```python
from build123d import *

# Parameters (mm, degrees)
PAD_DEPTH       = 33
POCKET_DEPTH    = 28
PAD001_DEPTH    = 4
SKETCH003_R     = 2.75
PAD002_DEPTH    = 5
SKETCH004_R     = 3.125
PAD003_DEPTH    = 3
FILLET_R        = 34
FILLET001_R     = 12
FILLET002_R     = 2
CHAMFER_SIZE    = 1
CHAMFER001_SIZE = 1
CHAMFER002_SIZE = 1


with BuildPart() as part:
    # Sketch → Pad (new body)
    with BuildSketch(Plane.XY):
        Polygon((-30, 0), (30, 0), (30, -51.038384), (0, -120), (-30, -51.038384), align=None)
    extrude(amount=PAD_DEPTH)

    # Sketch001 (on Face7 of Pad) → Pocket (cut)
    with BuildSketch(Plane.XY.offset(33)):
        Polygon((-22.25, 3.29609), (22.25, 3.29609), (22.25, -49.798735), (0, -100), (-22.25, -49.798735), align=None)
    extrude(amount=-POCKET_DEPTH, mode=Mode.SUBTRACT)

    # Sketch002 (on Face4 of Pocket) → Pad001 (join)
    with BuildSketch(Plane.XY.offset(33)):
        Polygon((-30, 0), (30, 0), (30, -51.038384), (0, -120), (-30, -51.038384), align=None)
    extrude(amount=-PAD001_DEPTH)

    # Sketch003 (on Face2 of Pad001) → Pad002 (join)
    with BuildSketch(Plane(origin=(0, 0, 0), x_dir=(1, 0, 0), z_dir=(0, 0, -1))):
        with Locations((-12.7, 22.314992)):
            Circle(SKETCH003_R)
        with Locations((12.7, 22.314992)):
            Circle(SKETCH003_R)
        with Locations((-12.7, 47.714992)):
            Circle(SKETCH003_R)
        with Locations((12.7, 47.714992)):
            Circle(SKETCH003_R)
    extrude(amount=PAD002_DEPTH)

    # Sketch004 (on Face25 of Pad002) → Pad003 (join)
    with BuildSketch(Plane(origin=(0, 0, -5), x_dir=(1, 0, 0), z_dir=(0, 0, -1))):
        with Locations((12.7, 47.714992)):
            Circle(SKETCH004_R)
        with Locations((-12.7, 47.714992)):
            Circle(SKETCH004_R)
        with Locations((-12.7, 22.314992)):
            Circle(SKETCH004_R)
        with Locations((12.7, 22.314992)):
            Circle(SKETCH004_R)
    extrude(amount=PAD003_DEPTH)

    # Fillet
    fillet_edges = [part.edges().sort_by_distance(p)[0] for p in [
        (30, -51.038384, 14.5),
        (-30, -51.038384, 14.5),
    ]]
    fillet(fillet_edges, radius=FILLET_R)

    # Fillet001
    fillet001_edges = [part.edges().sort_by_distance(p)[0] for p in [
        (0, -120, 14.5),
    ]]
    fillet(fillet001_edges, radius=FILLET001_R)

    # Fillet002
    fillet002_edges = [part.edges().sort_by_distance(p)[0] for p in [
        (-30, 0, 14.5),
        (30, 0, 14.5),
    ]]
    fillet(fillet002_edges, radius=FILLET002_R)

    # Chamfer
    chamfer_edges = [part.edges().sort_by_distance(p)[0] for p in [
        (30, -22.981604, 33),
    ]]
    chamfer(chamfer_edges, length=CHAMFER_SIZE)

    # Chamfer001
    chamfer001_edges = [part.edges().sort_by_distance(p)[0] for p in [
        (0, 0, 0),
    ]]
    chamfer(chamfer001_edges, length=CHAMFER001_SIZE)

    # Chamfer002
    chamfer002_edges = [part.edges().sort_by_distance(p)[0] for p in [
        (-15.825, -22.314992, -8),
        (9.575, -22.314992, -8),
        (9.575, -47.714992, -8),
        (-15.825, -47.714992, -8),
    ]]
    chamfer(chamfer002_edges, length=CHAMFER002_SIZE)


solid = part.part
```
Design review of the part built by this model. Coordinates are the model's own, in mm. A direction names the side the tool comes from. Round coordinates to 2 decimals unless told otherwise and drop trailing zeros. Write each loop counter-clockwise with the first axis right and the second up, starting at its lowest first coordinate (ties: lowest second). Pieces come first, ordered by that corner, then holes.
Item 1: For faces 5 (the flat face through (0, 0, 30)), 6 (the flat face through (0, -38, 5)), list the 3-axis set-ups (+Z, -Z, +X, -X, +Y, -Y) from which the entire face can be reached by the end or side of a thin tool; tool diameter is ignored.
Item 2: We need section D-D on y = -88. Write out the cut boundary in (x, z).
Item 3: We need section A-A on y = -36.5. Write out the cut boundary in (x, z), and give its area (3 significant figures).
Item 4: Clearance check with flat-ended pins moving along their axes: pin 1 Ø22 at (x, y) = (3, -45.5) entering from -Z; pin 2 Ø1 at (x, z) = (11, 6.5) entering from +Y; pin 3 Ø1.5 at (x, y) = (-2.5, -41.5) entering from -Z; pin 4 Ø5 at (y, z) = (-69.5, 6.5) entering from -X. State where each tip first meets the part, or that it passes through.
Item 5: For probe 1 along Z at (x, y) = (10, -24); probe 2 along X at (y, z) = (-37.5, 19); probe 3 along X at (y, z) = (-93, 9.5), list the stretches that pass through material, from the lowest coordinate up.
Item 6: The part is to be moulded in two halves that separate along Y. For faces 1 (the cylindrical face through (-13.06, -50.44, -2.46)), 2 (the flat face through (13, -48, -8)), 3 (the flat face through (18.752, -75.659, 0.507)), 4 (the cylindrical face through (10.52, -20.64, -2.46)), say which applies: +Y half, -Y half, draft (parallel to the pull), parting line (faces both ways), or undercut.
Item 7: We need section B-B on z = 25.5. Write out the cut boundary in (x, y), and give its area (3 significant figures).
Item 8: We need section C-C on x = -20.5. Write out the cut boundary in (y, z), and give its area (3 significant figures).
Returned:
1. face 5: +Z, -Z, +X, -X, +Y
1. face 6: +Y
2. outline: (-13.92, 1) - (-12.83, 0) - (12.83, 0) - (13.92, 1) - (13.92, 32) - (12.83, 33) - (-12.83, 33) - (-13.92, 32) - close; hole (-5.32, 5) - (5.32, 5) - (5.32, 29) - (-5.32, 29) - close
3. outline: (-30, 1) - (-29, 0) - (29, 0) - (30, 1) - (30, 32) - (29, 33) - (-29, 33) - (-30, 32) - close; hole (-22.25, 5) - (22.25, 5) - (22.25, 29) - (-22.25, 29) - close
3. area: 910 mm2
4. pin 1: stops at z = -8
4. pin 2: stops at y = -74.05
4. pin 3: stops at z = 0
4. pin 4: stops at x = -23.06
5. probe 1: z = 0 to 5, 29 to 33
5. probe 2: x = -30 to -22.25, 22.25 to 30
5. probe 3: x = -11.75 to -3.1, 3.1 to 11.75
6. face 1: undercut
6. face 2: draft
6. face 3: -Y half
6. face 4: undercut
7. outline: (-30, -43.96) arc R34 ccw to (-27.18, -57.53) - (-11, -94.71) arc R12 ccw to (11, -94.71) - (27.18, -57.53) arc R34 ccw to (30, -43.96) - (30, -2) arc R2 ccw to (28, 0) - (22.25, 0) - (22.25, -49.8) - (0, -100) - (-22.25, -49.8) - (-22.25, 0) - (-28, 0) arc R2 ccw to (-30, -2) - close
7. area: 1,630 mm2
8. outline: (-72.88, 1) - (-70.37, 0) - (-1, 0) - (0, 1) - (0, 5) - (-53.75, 5) - (-53.75, 29) - (0, 29) - (0, 32) - (-1, 33) - (-70.37, 33) - (-72.88, 32) - close
8. area: 1,110 mm2
